Design review of the part built by this model. Coordinates are the model's own, in mm. A direction names the side the tool comes from. Coordinates: 2 decimals unless noted, no trailing zeros. Order: outer loops, then holes, each group sorted by start corner. A loop starts at its lowest first (then second) coordinate and runs counter-clockwise, first axis right, second up. Notation, with made-up numbers: (-18, 58.5) - (21, 58.5) arc R37 ccw to (21, 95.5) - close; hole circle Ø4 at (17, -32.75). An arc over 180 degrees is marked (long way). Write item = value, one per line. Start each with the question number.
```python
from build123d import *

# Parameters (mm, degrees)
SKETCH014_W     = 12.3
SKETCH014_H     = 209.55
PAD003_DEPTH    = 25.4
SKETCH015_W     = 12.3
SKETCH015_H     = 6.35
POCKET011_DEPTH = 12.7
SKETCH016_R     = 2
POCKET012_DEPTH = 10
SKETCH017_W     = 6.35
SKETCH017_H     = 50.8
POCKET013_DEPTH = 25.401
SKETCH018_R     = 3
POCKET014_DEPTH = 5.951
CHAMFER003_SIZE = 1.5


with BuildPart() as part:
    # Sketch014 → Pad003 (new body)
    with BuildSketch(Plane.XY):
        with Locations((-82.55, 111.125)):
            Rectangle(SKETCH014_W, SKETCH014_H)
    extrude(amount=PAD003_DEPTH)

    # Sketch015 (on Face5 of Pad003) → Pocket011 (cut)
    with BuildSketch(Plane(origin=(0, 0, 0), x_dir=(1, 0, 0), z_dir=(0, 0, -1))):
        with Locations((-82.55, -9.525)):
            Rectangle(SKETCH015_W, SKETCH015_H)
    extrude(amount=-POCKET011_DEPTH, mode=Mode.SUBTRACT)

    # Sketch016 (on Face1 of Pocket011) → Pocket012 (cut)
    with BuildSketch(Plane.XZ.offset(-6.35)):
        with Locations((-82.55, 19.05)):
            Circle(SKETCH016_R)
    extrude(amount=-POCKET012_DEPTH, mode=Mode.SUBTRACT)

    # Sketch017 (on Face5 of Pocket012) → Pocket013 (cut, through all)
    with BuildSketch(Plane.XY.offset(25.4)):
        with Locations((-79.575, 190.5)):
            Rectangle(SKETCH017_W, SKETCH017_H)
    extrude(amount=-POCKET013_DEPTH, mode=Mode.SUBTRACT)

    # Sketch018 (on Face11 of Pocket013) → Pocket014 (cut, through all)
    with BuildSketch(Plane.YZ.offset(-82.75)):
        with Locations((190.5, 12.7)):
            Circle(SKETCH018_R)
        with Locations((209.9, 12.7)):
            Circle(SKETCH018_R)
    extrude(amount=-POCKET014_DEPTH, mode=Mode.SUBTRACT)

    # Chamfer003
    chamfer003_edges = [part.edges().sort_by_distance(p)[0] for p in [
        (-88.7, 187.5, 12.7),
        (-88.7, 206.9, 12.7),
    ]]
    chamfer(chamfer003_edges, length=CHAMFER003_SIZE)


solid = part.part
```
Item 1: Add section B-B on z = 5. Give the boundary of the cut face in (x, y), plus the area to 3 significant figures.
Item 2: For faces 1 (the flat face through (-83, 16.35, 19)), 2 (the flat face through (-83, 9, 12.7)), 3 (the flat face through (-80, 165.1, 13)), list the 3-axis set-ups (+Z, -Z, +X, -X, +Y, -Y) from which the entire face can be reached by the end or side of a thin tool; tool diameter is ignored.
Item 3: For P1, Ø1.9, axis at x = -85, y = 10, coming from the -Z side; P2, Ø5, axis at y = 190.5, z = 12.7, coming from the -X side; P3, Ø5, axis at x = -78.5, z = 18, coming from the +Y side; P4, Ø3.5, axis at x = -83, z = 6, coming from the -Y side, all flat-tipped, find the tip position at first contact; note any pin that passes through.
Item 4: Mouldability with a two-part tool opening along Z and no side actions: class faces 4 (the cylindrical face through (-84.548, 11.28, 19.138)), 5 (the flat face through (-83, 113, 25.4)), 6 (the flat face through (-82.75, 190, 16)) as +Z half, -Z half, draft (parallel to the pull), parting line (faces both ways), or undercut.
Item 5: For line 1 (Z direction, x = -82.55, y = 13.25); line 2 (Z direction, x = -83.8, y = 190.5); line 3 (X direction, y = 205, z = 9), list the stretches that pass through material, from the lowest coordinate up.
Item 6: Add section A-A on y = 209.9. Give the boundary of the cut face in (x, z), plus the area to 3 significant figures.
Worked out:
q1.outline = (-88.7, 12.7) - (-76.4, 12.7) - (-76.4, 165.1) - (-82.75, 165.1) - (-82.75, 215.9) - (-88.7, 215.9) - close
q1.area = 2,180 mm2
q2.face_1 = -Y
q2.face_2 = -Z, +X, -X, -Y
q2.face_3 = +Z, -Z, +X, +Y
q3.P1 = 12.7
q3.P2 = through
q3.P3 = 165.1
q3.P4 = 12.7
q4.face_4 = undercut
q4.face_5 = +Z half
q4.face_6 = draft
q5.line_1 = 0 to 17.05, 21.05 to 25.4
q5.line_2 = 0 to 9.7, 15.7 to 25.4
q5.line_3 = -88.7 to -82.75
q6.outline = (-88.7, 0) - (-82.75, 0) - (-82.75, 9.7) - (-87.2, 9.7) - (-88.7, 8.2) - close; (-88.7, 17.2) - (-87.2, 15.7) - (-82.75, 15.7) - (-82.75, 25.4) - (-88.7, 25.4) - close
q6.area = 113 mm2
